from build123d import *

# Parameters (mm, degrees)
SKETCH1_R           = 91.44
SKETCH1_R_2         = 78.74
BOSS_EXTRUDE1_DEPTH = 50.8
CHAMFER1_SIZE       = 2.54
SKETCH2_W           = 16.258151814
SKETCH2_H           = 87.529352209
CUT_EXTRUDE1_DEPTH  = 127
CIRPATTERN1_COUNT   = 4
SKETCH3_R           = 3.2639
CUT_EXTRUDE2_DEPTH  = 204.799389413
CIRPATTERN2_COUNT   = 4


with BuildPart() as part:
    # Sketch1 → Boss-Extrude1 (new body)
    with BuildSketch(Plane(origin=(0, 0, 0), x_dir=(1, 0, 0), z_dir=(0, 1, 0))):
        with Locations(Location((0, 0, 0), (0, 0, 270))):
            Circle(SKETCH1_R)
        with Locations(Location((0, 0, 0), (0, 0, 270))):
            Circle(SKETCH1_R_2, mode=Mode.SUBTRACT)
    extrude(amount=BOSS_EXTRUDE1_DEPTH)

    # Chamfer1
    chamfer1_edges = [part.edges().sort_by_distance(p)[0] for p in [
        (0, 0, -91.44),
        (0, 50.8, -91.44),
        (0, 0, -78.74),
    ]]
    chamfer(chamfer1_edges, length=CHAMFER1_SIZE)

    # Sketch2 → Cut-Extrude1 (cut, symmetric)
    with BuildSketch(Plane.XY):
        with Locations((96.394075907, 25.589048277)):
            Rectangle(SKETCH2_W, SKETCH2_H)
    cut_extrude1 = extrude(amount=CUT_EXTRUDE1_DEPTH, both=True, mode=Mode.SUBTRACT)

    # CirPattern1: Cut-Extrude1 ×4 about axis
    cirpattern1_axis = Axis((0, 0, 0), (0, 1, 0))
    for i in range(1, CIRPATTERN1_COUNT):
        add(cut_extrude1.rotate(cirpattern1_axis, i * 360 / CIRPATTERN1_COUNT), mode=Mode.SUBTRACT)

    # Sketch3 → Cut-Extrude2 (cut, through all)
    with BuildSketch(Plane(origin=(0, 0, -88.265), x_dir=(-1, 0, 0), z_dir=(0, 0, -1))):
        with Locations((3.65e-06, 25.4)):
            Circle(SKETCH3_R)
    cut_extrude2 = extrude(amount=-CUT_EXTRUDE2_DEPTH, mode=Mode.SUBTRACT)

    # CirPattern2: Cut-Extrude2 ×4 about axis
    cirpattern2_axis = Axis((0, 50.8, 0), (0, 1, 0))
    for i in range(1, CIRPATTERN2_COUNT):
        add(cut_extrude2.rotate(cirpattern2_axis, i * 360 / CIRPATTERN2_COUNT), mode=Mode.SUBTRACT)


solid = part.part
The listing builds one solid part. Answer for the finished solid, in the listing's coordinates (mm). Give positions to 0.01 mm unless a question says otherwise; leave off trailing zeros. Order: outer loops, then holes, each group sorted by start corner. A loop starts at its lowest first (then second) coordinate and runs counter-clockwise, first axis right, second up. Notation, with made-up numbers: (14, 8) -> (62, 8) arc R24 ccw to (62, 36) -> close; hole circle Ø1 at (4.5, -16.5). An arc over 180 degrees is marked (long way). Put each result on its own line as item: value.
Item 1: Given P1, Ø5, axis at y = 23.5, z = 44, coming from the -X side; P2, Ø3, axis at y = 6.5, z = 58.5, coming from the +X side; P3, Ø4, axis at x = 62, z = 68.5, coming from the +Y side, each flat-ended and moving along its own axis, determine where each tip first touches the part or whether it passes through.
Established:
P1: stops at x = -81.48
P2: stops at x = 71.5
P3: stops at y = 49.31
Item 2: A cutting plane is placed at A-A on y = 25.4. Give the vertices of the cut face in (x, z) (3 decimals).
Established:
outline: (-88.265, -23.886) arc R91.44 ccw to (-23.886, -88.265) -> (-3.264, -88.265) -> (-3.264, -78.672) arc R78.74 cw to (-78.672, -3.264) -> (-88.265, -3.264) -> close; (-88.265, 3.264) -> (-78.672, 3.264) arc R78.74 cw to (-3.264, 78.672) -> (-3.264, 88.265) -> (-23.886, 88.265) arc R91.44 ccw to (-88.265, 23.886) -> close; (3.264, -88.265) -> (23.886, -88.265) arc R91.44 ccw to (88.265, -23.886) -> (88.265, -3.264) -> (78.672, -3.264) arc R78.74 cw to (3.264, -78.672) -> close; (3.264, 78.672) arc R78.74 cw to (78.672, 3.264) -> (88.265, 3.264) -> (88.265, 23.886) arc R91.44 ccw to (23.886, 88.265) -> (3.264, 88.265) -> close
Item 3: Straight lines are drawn through the part: line 1 (X direction, y = 14.5, z = 0) (3 decimals); line 2 (Z direction, x = -63, y = 4). For each, find the intervals that lie inside material, in ascending order.
Established:
line 1: x = -88.265 to -78.74, 78.74 to 88.265
line 2: z = -66.27 to -47.23, 47.23 to 66.27
Item 4: For a pull along X with two mould halves and no side action, classify faces 1 (the face through (-65.13, 25.08, 64.18)), 2 (the face through (-72, 0, 39)), 3 (the face through (-76.868, 26.332, -17.069)) as released by +X, released by -X, zero draft, split by the parting line, or undercut.
Established:
face 1: released by -X
face 2: zero draft
face 3: undercut
